```python
from build123d import *

# Parameters (mm, degrees)
F1_ANGLE = 180
F2_W     = 30.71798
F2_H     = 26.843641
F3_DEPTH = 100


with BuildPart() as f1:
    # F0 (on Right) → F1 (revolve, symmetric)
    with BuildSketch(Plane.YZ) as f1_sk:
        Polygon((-15, -70.817309), (0, -70.817309), (0, -68.317309), (-12.5, -68.317309), (-12.500003, 20.655008), (-15.000003, 20.655008), (-15.000003, -6.844992), (-45.000003, -6.844992), (-63.529334, -29.72469), (-61.58654, -31.298079), (-45.000003, -10.817309), (-15, -10.817309), align=None)
    revolve(axis=Axis((0, 0, -69.567309), (0, 0, 1)), revolution_arc=F1_ANGLE / 2)
    revolve(f1_sk.sketch, axis=Axis((0, 0, -69.567309), (0, 0, -1)), revolution_arc=F1_ANGLE / 2)

    # F2 (on Front) → F3 (cut)
    with BuildSketch(Plane.XZ):
        with Locations((-0.268487, 7.287501)):
            Rectangle(F2_W, F2_H)
    extrude(amount=F3_DEPTH, mode=Mode.SUBTRACT)


solid = f1.part
```
Read the model definition and answer for the solid it produces. Units are mm, in the model's axes. A direction names the side the tool comes from. Give positions to 0.01 mm unless a question says otherwise; leave off trailing zeros. Order: outer loops, then holes, each group sorted by start corner. A loop starts at its lowest first (then second) coordinate and runs counter-clockwise, first axis right, second up.
(1) Given pin 1 (6 mm diameter, centred on x = 41, y = -35.5, fed in from -Z); pin 2 (1 mm diameter, centred on x = -7.5, z = -48, fed in from -Y); pin 3 (1 mm diameter, centred on x = 1, y = -19, fed in from -Z), each flat-ended and moving along its own axis, determine where each tip first touches the part or whether it passes through.
(2) For a pull along Y with two mould halves and no side action, classify faces 1 (the flat face through (-1, -23, -6.845)), 2 (the cylindrical face through (0.33, -14.996, -6.495)), 3 (the cylindrical face through (0, -15, -41)) as released by +Y, released by -Y, zero draft, split by the parting line, or undercut.
(3) Find section C-C (z = -44.5). Give the vertices of the cut face in (x, y), plus the area to 3 significant figures.
(4) Find section B-B (z = -26). Give the vertices of the cut face in (x, y).
(5) For faces 4 (the conical face through (1.02, -46.15, -8.28)), 5 (the flat face through (0, -5, -68.317)), 6 (the flat face through (-1, -22, -10.817)), determine the directions among +Z, -Z, +X, -X, +Y, -Y from which every point of the face is accessible in a straight line to the end or side of a thin tool.
(6) Straight lines are drawn through the part: L1, parallel to Z at x = -35.5, y = -11 (3 decimals); L2, parallel to X at y = -4, z = -48; L3, parallel to Y at x = 3, z = -27.5. For each, find the intervals that lie inside material, in ascending order.
(7) Find section A-A (x = 0). Give the vertices of the cut face in (y, z) (3 decimals), plus the area to 3 significant figures.
Result sheet:
1. pin 1: stops at z = -25.92
1. pin 2: stops at y = -13.27
1. pin 3: stops at z = -10.82
2. face 1: zero draft
2. face 2: released by -Y
2. face 3: undercut
3. outline: (-15, 0) arc R15 ccw to (15, 0) - (12.5, 0) arc R12.5 cw to (-12.5, 0) - close
3. area: 108 mm2
4. outline: (-60.51, 0) arc R60.51 ccw to (60.51, 0) - (57.3, 0) arc R57.3 cw to (-57.3, 0) - close; (-15, 0) arc R15 ccw to (15, 0) - (12.5, 0) arc R12.5 cw to (-12.5, 0) - close
5. face 4: +Z, -Y
5. face 5: +Z, +Y
5. face 6: -Z
6. L1: z = -10.817 to -6.845
6. L2: x = -14.46 to -11.84, 11.84 to 14.46
6. L3: y = -61.65 to -58.43, -14.7 to -12.13
7. outline: (-63.529, -29.725) - (-61.587, -31.298) - (-45, -10.817) - (-15, -10.817) - (-15, -70.817) - (0, -70.817) - (0, -68.317) - (-12.5, -68.317) - (-12.5, -6.134) - (-15, -6.134) - (-15, -6.845) - (-45, -6.845) - close
7. area: 382 mm2
